from build123d import *

# Parameters (mm, degrees)
MODEL_R                 = 1.5
MODEL_W                 = 3
MODEL_H                 = 3
SALIENTE_EXTRUIR1_DEPTH = 3


with BuildPart() as part:
    # Model → Saliente-Extruir1 (new body)
    with BuildSketch(Plane.XY):
        with BuildLine():
            Line((13.608524471, 199.498543913), (49.608524471, 199.498543913))
            ThreePointArc((49.608524471, 199.498543913), (52.790504986, 200.816563398), (54.108524471, 203.998543913))
            Line((54.108524471, 203.998543913), (54.108524471, 293.998543913))
            ThreePointArc((54.108524471, 293.998543913), (52.790504986, 297.180524429), (49.608524471, 298.498543913))
            Line((49.608524471, 298.498543913), (13.608524471, 298.498543913))
            ThreePointArc((13.608524471, 298.498543913), (10.426543955, 297.180524429), (9.108524471, 293.998543913))
            Line((9.108524471, 293.998543913), (9.108524471, 203.998543913))
            ThreePointArc((9.108524471, 203.998543913), (10.426543955, 200.816563398), (13.608524471, 199.498543913))
        make_face()
        with Locations((45.108524471, 266.998543913)):
            Circle(MODEL_R, mode=Mode.SUBTRACT)
        with Locations((18.108524471, 266.998543913)):
            Circle(MODEL_R, mode=Mode.SUBTRACT)
        with Locations((49.608524471, 262.498543913)):
            Circle(MODEL_R, mode=Mode.SUBTRACT)
        with Locations((49.608524471, 271.498543913)):
            Circle(MODEL_R, mode=Mode.SUBTRACT)
        with Locations((13.608524471, 262.498543913)):
            Circle(MODEL_R, mode=Mode.SUBTRACT)
        with Locations((13.608524471, 271.498543913)):
            Circle(MODEL_R, mode=Mode.SUBTRACT)
        with Locations((49.608524471, 293.998543913)):
            Rectangle(MODEL_W, MODEL_H, mode=Mode.SUBTRACT)
        with Locations((49.608524471, 284.998543913)):
            Rectangle(MODEL_W, MODEL_H, mode=Mode.SUBTRACT)
        with Locations((49.608524471, 275.998543913)):
            Rectangle(MODEL_W, MODEL_H, mode=Mode.SUBTRACT)
        with Locations((49.608524471, 266.998543913)):
            Rectangle(MODEL_W, MODEL_H, mode=Mode.SUBTRACT)
        with Locations((49.608524471, 257.998543913)):
            Rectangle(MODEL_W, MODEL_H, mode=Mode.SUBTRACT)
        with Locations((49.608524471, 248.998543913)):
            Rectangle(MODEL_W, MODEL_H, mode=Mode.SUBTRACT)
        with Locations((49.608524471, 239.998543913)):
            Rectangle(MODEL_W, MODEL_H, mode=Mode.SUBTRACT)
        with Locations((49.608524471, 230.998543913)):
            Rectangle(MODEL_W, MODEL_H, mode=Mode.SUBTRACT)
        with Locations((49.608524471, 221.998543913)):
            Rectangle(MODEL_W, MODEL_H, mode=Mode.SUBTRACT)
        with Locations((49.608524471, 212.998543913)):
            Rectangle(MODEL_W, MODEL_H, mode=Mode.SUBTRACT)
        with Locations((49.608524471, 203.998543913)):
            Rectangle(MODEL_W, MODEL_H, mode=Mode.SUBTRACT)
        with Locations((13.608524471, 293.998543913)):
            Rectangle(MODEL_W, MODEL_H, mode=Mode.SUBTRACT)
        with Locations((13.608524471, 284.998543913)):
            Rectangle(MODEL_W, MODEL_H, mode=Mode.SUBTRACT)
        with Locations((13.608524471, 275.998543913)):
            Rectangle(MODEL_W, MODEL_H, mode=Mode.SUBTRACT)
        with Locations((13.608524471, 266.998543913)):
            Rectangle(MODEL_W, MODEL_H, mode=Mode.SUBTRACT)
        with Locations((13.608524471, 257.998543913)):
            Rectangle(MODEL_W, MODEL_H, mode=Mode.SUBTRACT)
        with Locations((13.608524471, 248.998543913)):
            Rectangle(MODEL_W, MODEL_H, mode=Mode.SUBTRACT)
        with Locations((13.608524471, 239.998543913)):
            Rectangle(MODEL_W, MODEL_H, mode=Mode.SUBTRACT)
        with Locations((13.608524471, 230.998543913)):
            Rectangle(MODEL_W, MODEL_H, mode=Mode.SUBTRACT)
        with Locations((13.608524471, 221.998543913)):
            Rectangle(MODEL_W, MODEL_H, mode=Mode.SUBTRACT)
        with Locations((13.608524471, 212.998543913)):
            Rectangle(MODEL_W, MODEL_H, mode=Mode.SUBTRACT)
        with Locations((13.608524471, 203.998543913)):
            Rectangle(MODEL_W, MODEL_H, mode=Mode.SUBTRACT)
        with Locations((40.608524471, 203.998543913)):
            Rectangle(MODEL_W, MODEL_H, mode=Mode.SUBTRACT)
        with Locations((22.608524471, 203.998543913)):
            Rectangle(MODEL_W, MODEL_H, mode=Mode.SUBTRACT)
        with Locations((31.608524471, 203.998543913)):
            Rectangle(MODEL_W, MODEL_H, mode=Mode.SUBTRACT)
        with Locations((40.608524471, 221.998543913)):
            Rectangle(MODEL_W, MODEL_H, mode=Mode.SUBTRACT)
        with Locations((22.608524471, 221.998543913)):
            Rectangle(MODEL_W, MODEL_H, mode=Mode.SUBTRACT)
        with Locations((31.608524471, 221.998543913)):
            Rectangle(MODEL_W, MODEL_H, mode=Mode.SUBTRACT)
        with Locations((40.608524471, 212.998543913)):
            Rectangle(MODEL_W, MODEL_H, mode=Mode.SUBTRACT)
        with Locations((22.608524471, 212.998543913)):
            Rectangle(MODEL_W, MODEL_H, mode=Mode.SUBTRACT)
        with Locations((31.608524471, 212.998543913)):
            Rectangle(MODEL_W, MODEL_H, mode=Mode.SUBTRACT)
        with Locations((40.608524471, 293.998543913)):
            Rectangle(MODEL_W, MODEL_H, mode=Mode.SUBTRACT)
        with Locations((22.608524471, 293.998543913)):
            Rectangle(MODEL_W, MODEL_H, mode=Mode.SUBTRACT)
        with Locations((31.608524471, 293.998543913)):
            Rectangle(MODEL_W, MODEL_H, mode=Mode.SUBTRACT)
        with Locations((40.608524471, 284.998543913)):
            Rectangle(MODEL_W, MODEL_H, mode=Mode.SUBTRACT)
        with Locations((22.608524471, 284.998543913)):
            Rectangle(MODEL_W, MODEL_H, mode=Mode.SUBTRACT)
        with Locations((40.608524471, 230.998543913)):
            Rectangle(MODEL_W, MODEL_H, mode=Mode.SUBTRACT)
        with Locations((22.608524471, 230.998543913)):
            Rectangle(MODEL_W, MODEL_H, mode=Mode.SUBTRACT)
        with Locations((31.608524471, 230.998543913)):
            Rectangle(MODEL_W, MODEL_H, mode=Mode.SUBTRACT)
        with Locations((31.608524471, 284.998543913)):
            Rectangle(MODEL_W, MODEL_H, mode=Mode.SUBTRACT)
        with BuildLine():
            Line((21.508214184, 276.698579599), (21.508214184, 236.948579599))
            ThreePointArc((21.508214184, 236.948579599), (21.654660793, 236.595026209), (22.008214184, 236.448579599))
            Line((22.008214184, 236.448579599), (41.208214184, 236.448579599))
            ThreePointArc((41.208214184, 236.448579599), (41.561767574, 236.595026209), (41.708214184, 236.948579599))
            Line((41.708214184, 236.948579599), (41.708214184, 276.698579599))
            ThreePointArc((41.708214184, 276.698579599), (41.561767574, 277.05213299), (41.208214184, 277.198579599))
            Line((41.208214184, 277.198579599), (36.608214184, 277.198579599))
            ThreePointArc((36.608214184, 277.198579599), (35.901107403, 277.491472818), (35.608214184, 278.198579599))
            Line((35.608214184, 278.198579599), (35.608214184, 280.198579599))
            ThreePointArc((35.608214184, 280.198579599), (35.315320965, 280.905686381), (34.608214184, 281.198579599))
            Line((34.608214184, 281.198579599), (28.608214184, 281.198579599))
            ThreePointArc((28.608214184, 281.198579599), (27.901107403, 280.905686381), (27.608214184, 280.198579599))
            Line((27.608214184, 280.198579599), (27.608214184, 278.198579599))
            ThreePointArc((27.608214184, 278.198579599), (27.315320965, 277.491472818), (26.608214184, 277.198579599))
            Line((26.608214184, 277.198579599), (22.008214184, 277.198579599))
            ThreePointArc((22.008214184, 277.198579599), (21.654660793, 277.05213299), (21.508214184, 276.698579599))
        make_face(mode=Mode.SUBTRACT)
    extrude(amount=SALIENTE_EXTRUIR1_DEPTH)


solid = part.part
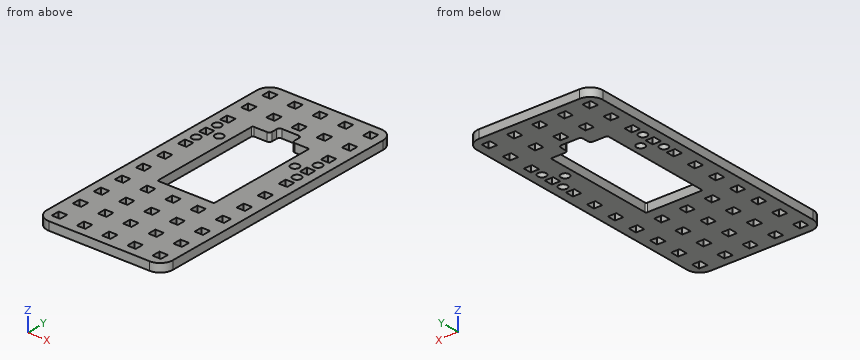
CAD build for the part. Positions are in the model's coordinates, mm. Coordinates: 2 decimals unless noted, no trailing zeros. Loops run counter-clockwise (first coordinate to the right, second up) from the corner with the lowest first, then second, coordinate; pieces in that order, holes last. Notation, with made-up numbers: (66.25, 25.25) - (111.25, 25.25) arc R23 ccw to (111.25, 58.25) - close; hole circle Ø11 at (88.25, -11). An arc over 180 degrees is marked (long way). Write item = value, one per line. Start each with the question number.
Q1. Cut at B-B, the plane y = 258. List the corners of the cut face in (x, z).
Q2. Cut at A-A, the plane y = 245. List the corners of the cut face in (x, z), then the cut area to 3 significant figures.
Q3. Drill centre lines: L1, parallel to X at y = 262.5, z = 2.3; L2, parallel to X at y = 285, z = 2.65; L3, parallel to Y at x = 29, z = 2.45. Where is each one in solid material? Low to high.
Q4. Cut at C-C, the plane x = 17.5. List the corners of the cut face in (y, z), then the cut area to 3 significant figures.
Q5. Flat gauge pins, fed straight in: pin 1 Ø0.9 at (x, z) = (13, 1) entering from -Y; pin 2 Ø1 at (x, y) = (29, 278.5) entering from -Z. Where does each tip first touch, or does it go through?
Q6. Cut at D-D, the plane z = 0.9. Give the number of separate pieces and of enclosed holes in the cut face, then the cut area to 3 significant figures.
Computed:
q1.outline = (9.11, 0) - (12.11, 0) - (12.11, 3) - (9.11, 3) - close; (15.11, 0) - (21.51, 0) - (21.51, 3) - (15.11, 3) - close; (41.71, 0) - (48.11, 0) - (48.11, 3) - (41.71, 3) - close; (51.11, 0) - (54.11, 0) - (54.11, 3) - (51.11, 3) - close
q2.outline = (9.11, 0) - (21.51, 0) - (21.51, 3) - (9.11, 3) - close; (41.71, 0) - (54.11, 0) - (54.11, 3) - (41.71, 3) - close
q2.area = 74.4 mm²
q3.L1 = 9.11 to 12.11, 15.11 to 21.51, 41.71 to 48.11, 51.11 to 54.11
q3.L2 = 9.11 to 12.11, 15.11 to 21.11, 24.11 to 30.11, 33.11 to 39.11, 42.11 to 48.11, 51.11 to 54.11
q3.L3 = 199.5 to 236.45, 281.2 to 298.5
q4.outline = (199.5, 0) - (265.63, 0) - (265.63, 3) - (199.5, 3) - close; (268.37, 0) - (298.5, 0) - (298.5, 3) - (268.37, 3) - close
q4.area = 289 mm²
q5.pin_1 = 199.5
q5.pin_2 = through
q6.separate_pieces = 1
q6.enclosed_holes = 47
q6.area = 3,180 mm²
